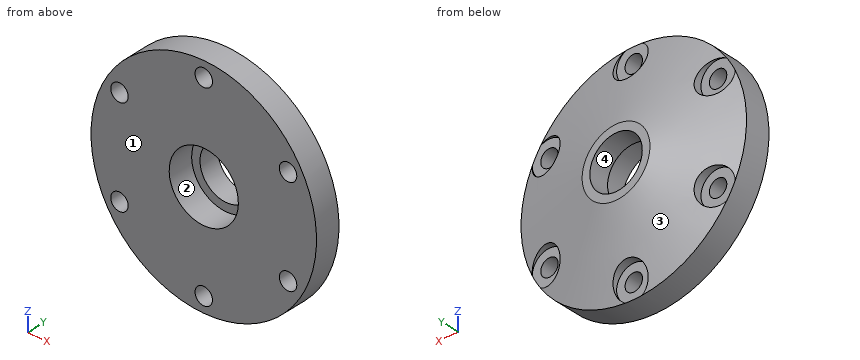
from build123d import *

# Parameters (mm, degrees)
M3_CLEARANCE_HOLE1_AT_2_COUNT  = 2
M3_CLEARANCE_HOLE1_AT_2_PITCH  = 19
M3_CLEARANCE_HOLE1_AT_3_COUNT  = 2
M3_CLEARANCE_HOLE1_AT_3_PITCH  = 32.908965344
M3_CLEARANCE_HOLE1_AT_4_COUNT  = 2
M3_CLEARANCE_HOLE1_AT_4_PITCH  = 38
M3_CLEARANCE_HOLE1_AT_5_COUNT  = 2
M3_CLEARANCE_HOLE1_AT_5_PITCH  = 32.908965344
M3_CLEARANCE_HOLE1_AT_6_COUNT  = 2
M3_CLEARANCE_HOLE1_AT_6_PITCH  = 19
M3_CLEARANCE_HOLE1_AT_7_COUNT  = 2
M3_CLEARANCE_HOLE1_AT_7_PITCH  = 19
CBORE_FOR_M3_SBHCS7_AT_2_COUNT = 2
CBORE_FOR_M3_SBHCS7_AT_2_PITCH = 19
CBORE_FOR_M3_SBHCS7_AT_3_COUNT = 2
CBORE_FOR_M3_SBHCS7_AT_3_PITCH = 32.908965344
CBORE_FOR_M3_SBHCS7_AT_4_COUNT = 2
CBORE_FOR_M3_SBHCS7_AT_4_PITCH = 38
CBORE_FOR_M3_SBHCS7_AT_5_COUNT = 2
CBORE_FOR_M3_SBHCS7_AT_5_PITCH = 32.908965344
CBORE_FOR_M3_SBHCS7_AT_6_COUNT = 2
CBORE_FOR_M3_SBHCS7_AT_6_PITCH = 19


with BuildPart() as part:
    # Sketch1 → Revolve1 (revolve)
    with BuildSketch(Plane.XY, mode=Mode.PRIVATE) as revolve1_sk:
        Polygon((5.12, 5), (5.12, 8.9453), (6.625, 8.9453), (22, 5), (22, 0), (6.75, 0), (6.75, 5), align=None)
    revolve(revolve1_sk.sketch.rotate(Axis((0, 0, 0), (0, 1, 0)), 90), axis=Axis((0, 0, 0), (0, 1, 0)))

    # Sketch3 → M3 Clearance Hole1 (revolve, cut)
    with BuildSketch(Plane(origin=(0, 5, -19), x_dir=(0, 0, 1), z_dir=(1, 0, 0))):
        Polygon((0, 0), (0, 6.021463052), (1.7, 5), (1.7, 0), align=None)
    m3_clearance_hole1 = revolve(axis=Axis((0, 11.35, -19), (0, -1, 0)), mode=Mode.SUBTRACT)

    # M3 Clearance Hole1 at 2: M3 Clearance Hole1 ×2
    with Locations(*[Vector(0.8660254037844387, 0, 0.49999999999999994) * (i * M3_CLEARANCE_HOLE1_AT_2_PITCH) for i in range(1, M3_CLEARANCE_HOLE1_AT_2_COUNT)]):
        add(m3_clearance_hole1, mode=Mode.SUBTRACT)

    # M3 Clearance Hole1 at 3: M3 Clearance Hole1 ×2
    with Locations(*[Vector(0.5000000000000001, 0, 0.8660254037844386) * (i * M3_CLEARANCE_HOLE1_AT_3_PITCH) for i in range(1, M3_CLEARANCE_HOLE1_AT_3_COUNT)]):
        add(m3_clearance_hole1, mode=Mode.SUBTRACT)

    # M3 Clearance Hole1 at 4: M3 Clearance Hole1 ×2
    with Locations(*[(0, 0, i * M3_CLEARANCE_HOLE1_AT_4_PITCH) for i in range(1, M3_CLEARANCE_HOLE1_AT_4_COUNT)]):
        add(m3_clearance_hole1, mode=Mode.SUBTRACT)

    # M3 Clearance Hole1 at 5: M3 Clearance Hole1 ×2
    with Locations(*[Vector(-0.49999999999999983, 0, 0.8660254037844388) * (i * M3_CLEARANCE_HOLE1_AT_5_PITCH) for i in range(1, M3_CLEARANCE_HOLE1_AT_5_COUNT)]):
        add(m3_clearance_hole1, mode=Mode.SUBTRACT)

    # M3 Clearance Hole1 at 6: M3 Clearance Hole1 ×2
    with Locations(*[Vector(-0.8660254037844387, 0, 0.4999999999999999) * (i * M3_CLEARANCE_HOLE1_AT_6_PITCH) for i in range(1, M3_CLEARANCE_HOLE1_AT_6_COUNT)]):
        add(m3_clearance_hole1, mode=Mode.SUBTRACT)

    # M3 Clearance Hole1 at 7: M3 Clearance Hole1 ×2
    with Locations(*[(0, 0, i * M3_CLEARANCE_HOLE1_AT_7_PITCH) for i in range(1, M3_CLEARANCE_HOLE1_AT_7_COUNT)]):
        add(m3_clearance_hole1, mode=Mode.SUBTRACT)

    # Sketch5 → CBORE for M3 SBHCS7 (revolve, cut)
    with BuildSketch(Plane(origin=(-16.454482672, 5, -9.5), x_dir=(0, 0, -1), z_dir=(1, 0, 0))):
        Polygon((0, 0), (0, 4.966763052), (1.7, 3.9453), (1.7, 1.65), (3.35, 1.65), (3.35, 0), align=None)
    cbore_for_m3_sbhcs7 = revolve(axis=Axis((-16.454482672, -1.35, -9.5), (0, 1, 0)), mode=Mode.SUBTRACT)

    # CBORE for M3 SBHCS7 at 2: CBORE for M3 SBHCS7 ×2
    with Locations(*[Vector(0.8660254037844387, 0, -0.4999999999999999) * (i * CBORE_FOR_M3_SBHCS7_AT_2_PITCH) for i in range(1, CBORE_FOR_M3_SBHCS7_AT_2_COUNT)]):
        add(cbore_for_m3_sbhcs7, mode=Mode.SUBTRACT)

    # CBORE for M3 SBHCS7 at 3: CBORE for M3 SBHCS7 ×2
    with Locations(*[(i * CBORE_FOR_M3_SBHCS7_AT_3_PITCH, 0, 0) for i in range(1, CBORE_FOR_M3_SBHCS7_AT_3_COUNT)]):
        add(cbore_for_m3_sbhcs7, mode=Mode.SUBTRACT)

    # CBORE for M3 SBHCS7 at 4: CBORE for M3 SBHCS7 ×2
    with Locations(*[Vector(0.8660254037844387, 0, 0.49999999999999994) * (i * CBORE_FOR_M3_SBHCS7_AT_4_PITCH) for i in range(1, CBORE_FOR_M3_SBHCS7_AT_4_COUNT)]):
        add(cbore_for_m3_sbhcs7, mode=Mode.SUBTRACT)

    # CBORE for M3 SBHCS7 at 5: CBORE for M3 SBHCS7 ×2
    with Locations(*[Vector(0.49999999999999994, 0, 0.8660254037844387) * (i * CBORE_FOR_M3_SBHCS7_AT_5_PITCH) for i in range(1, CBORE_FOR_M3_SBHCS7_AT_5_COUNT)]):
        add(cbore_for_m3_sbhcs7, mode=Mode.SUBTRACT)

    # CBORE for M3 SBHCS7 at 6: CBORE for M3 SBHCS7 ×2
    with Locations(*[(0, 0, i * CBORE_FOR_M3_SBHCS7_AT_6_PITCH) for i in range(1, CBORE_FOR_M3_SBHCS7_AT_6_COUNT)]):
        add(cbore_for_m3_sbhcs7, mode=Mode.SUBTRACT)


solid = part.part
Model file for the job. Use its own axes, mm. Face numbers are marked on the shaded views. Round coordinates to 2 decimals unless told otherwise and drop trailing zeros. Order: outer loops, then holes, each group sorted by start corner. A loop starts at its lowest first (then second) coordinate and runs counter-clockwise, first axis right, second up. Notation, with made-up numbers: M -38.5,13.25 L -24.5,13.25 A13 cw -24.5,37.25 Z; hole C 80,74 d3. An arc over 180 degrees is marked long. Write each question's results on one line, items separated by ' | '. Start each with the question number.
(1) Two-plate mould, pull along X, no slides. Class the marked faces 1, 2, 3 and 4: pulls with the +X half, pulls with the -X half, needs draft (parallel to the pull), parting line crosses it, or undercut.
(2) Saw through at C-C, the plane y = 7.75. Give the cut face in (x, z), then the cut area to 3 significant figures.
(3) Drop flat-ended pins along their axis: pin 1 (4 mm diameter, centred on x = 5, y = 2.5, fed in from +Z); pin 2 (10 mm diameter, centred on x = -7, z = 1.5, fed in from -Y); pin 3 (2.5 mm diameter, centred on x = 16.45, z = -9.5, fed in from +Y); pin 4 (5 mm diameter, centred on x = 1, z = -18.5, fed in from +Y). Give the stop position or say it passes through.
(4) Probe probe 1 along X at (y, z) = (1.35, -9.5); probe 2 along X at (y, z) = (2.4, 0); probe 3 along Z at (x, y) = (15, 2.75). List the from-to ranges inside material, lowest first. Write a range as from..to.
(5) Saw through at A-A, the plane z = 0. Give the cut face in (x, y) (3 decimals).
(6) Saw through at B-B, the plane y = 1. Give the cut face in (x, z).
Established:
1) face 1: needs draft | face 2: undercut | face 3: parting line crosses it | face 4: undercut
2) outline: C 0,0 d22.57; hole C 0,0 d10.24 | area: 318 mm^2
3) pin 1: stops at z = 21.79 | pin 2: stops at y = 0 | pin 3: passes through | pin 4: stops at y = 6.5
4) probe 1: x = -19.84..-18.15, -14.75..14.75, 18.15..19.84 | probe 2: x = -22..-6.75, 6.75..22 | probe 3: z = -16.09..-10.38, -8.62..8.62, 10.38..16.09
5) outline: M -22,0 L -6.75,0 L -6.75,5 L -5.12,5 L -5.12,8.945 L -6.625,8.945 L -22,5 Z; M 5.12,5 L 6.75,5 L 6.75,0 L 22,0 L 22,5 L 6.625,8.945 L 5.12,8.945 Z
6) outline: C 0,0 d44; hole C -16.45,-9.5 d3.4; hole C -16.45,9.5 d3.4; hole C 0,0 d13.5; hole C 0,-19 d3.4; hole C 0,19 d3.4; hole C 16.45,-9.5 d3.4; hole C 16.45,9.5 d3.4
